Design review of the part built by this model. Coordinates are the model's own, in mm. A direction names the side the tool comes from. Round coordinates to 2 decimals unless told otherwise and drop trailing zeros. Order: outer loops, then holes, each group sorted by start corner. A loop starts at its lowest first (then second) coordinate and runs counter-clockwise, first axis right, second up. Notation, with made-up numbers: M 10,40 L 38,40 A24 ccw 38,73 Z; hole C 35,67 d2. An arc over 180 degrees is marked long. Write each question's results on one line, items separated by ' | '. Start each with the question number.
Item 1: The part is to be moulded in two halves that separate along Y. For faces 1 (the flat face through (-1, 1.5, 6)), 2 (the cylindrical face through (51.64, -2.6, 4.31)), 3 (the flat face through (-1, 0, 2)), 4 (the cylindrical face through (-51.64, 2.6, 4.19)), say which applies: +Y half, -Y half, draft (parallel to the pull), parting line (faces both ways), or undercut.
Item 2: Wall thickness on line 1 (Y direction, x = -6, z = 3.25); line 2 (X direction, y = -0.75, z = 6); line 3 (Z direction, x = -46, y = 0.25): over which ranges is each line inside the solid? List them lowest first. Write a range as [from, to].
Item 3: Clearance check with a flat-ended pin moving along its axis: pin 1 (1.5 mm diameter, centred on x = -1, y = -0.5, fed in from +Z). State where the tip first meets the part, or that it passes through.
Item 4: Machinability: for faces 5 (the cylindrical face through (-51.64, -2.6, 4.31)), 6 (the flat face through (1, -1.5, 6)), which of the approach directions +Z, -Z, +X, -X, +Y, -Y give a long, thin tool a straight path to every point of the face, cutting with its end or side? Answer none if there is none.
Item 5: Take a section at B-B, the plane x = -31. Write out the cut boundary in (y, z).
Item 6: Take a section at A-A, the plane z = 7.5. Write out the cut boundary in (x, y).
```python
from build123d import *

# Parameters (mm, degrees)
F0_W     = 105
F0_H     = 7
F1_DEPTH = 2
F2_DEPTH = 10
F3_R     = 3
F4_R     = 1.5


with BuildPart() as f1:
    # F0 (on Top) → F1 (new body)
    with BuildSketch(Plane.XY):
        Rectangle(F0_W, F0_H)
        with BuildLine():
            ThreePointArc((-50.5, 0), (-50.0606601718, 1.0606601718), (-49, 1.5))
            Line((-49, 1.5), (49, 1.5))
            ThreePointArc((49, 1.5), (50.0606601718, 1.0606601718), (50.5, 0))
            ThreePointArc((50.5, 0), (50.0606601718, -1.0606601718), (49, -1.5))
            Line((49, -1.5), (-49, -1.5))
            ThreePointArc((-49, -1.5), (-50.0606601718, -1.0606601718), (-50.5, 0))
        make_face(mode=Mode.SUBTRACT)
        with BuildLine():
            Line((49, 1.5), (-49, 1.5))
            ThreePointArc((-49, 1.5), (-50.0606601718, 1.0606601718), (-50.5, 0))
            ThreePointArc((-50.5, 0), (-50.0606601718, -1.0606601718), (-49, -1.5))
            Line((-49, -1.5), (49, -1.5))
            ThreePointArc((49, -1.5), (50.0606601718, -1.0606601718), (50.5, 0))
            ThreePointArc((50.5, 0), (50.0606601718, 1.0606601718), (49, 1.5))
        make_face()
    extrude(amount=F1_DEPTH)

    # F0 (on Top) → F2 (join)
    with BuildSketch(Plane.XY):
        Rectangle(F0_W, F0_H)
        with BuildLine():
            ThreePointArc((-50.5, 0), (-50.0606601718, 1.0606601718), (-49, 1.5))
            Line((-49, 1.5), (49, 1.5))
            ThreePointArc((49, 1.5), (50.0606601718, 1.0606601718), (50.5, 0))
            ThreePointArc((50.5, 0), (50.0606601718, -1.0606601718), (49, -1.5))
            Line((49, -1.5), (-49, -1.5))
            ThreePointArc((-49, -1.5), (-50.0606601718, -1.0606601718), (-50.5, 0))
        make_face(mode=Mode.SUBTRACT)
    extrude(amount=F2_DEPTH)

    # F3
    f3_edges = [f1.edges().sort_by_distance(p)[0] for p in [
        (-52.5, -3.5, 5),
        (52.5, -3.5, 5),
        (52.5, 3.5, 5),
        (-52.5, 3.5, 5),
    ]]
    fillet(f3_edges, radius=F3_R)

    # F4
    f4_edges = [f1.edges().sort_by_distance(p)[0] for p in [
        (0, 3.5, 10),
    ]]
    fillet(f4_edges, radius=F4_R)


solid = f1.part
```
Results list:
1) face 1: undercut | face 2: -Y half | face 3: undercut | face 4: +Y half
2) line 1: [-3.5, -1.5], [1.5, 3.5] | line 2: [-52.49, -50.3], [50.3, 52.49] | line 3: [0, 2]
3) pin 1: z = 2
4) face 5: +Z, -Z, -X, -Y | face 6: +Z
5) outline: M -3.5,0 L 3.5,0 L 3.5,8.5 A1.5 ccw 2,10 L 1.5,10 L 1.5,2 L -1.5,2 L -1.5,10 L -2,10 A1.5 ccw -3.5,8.5 Z
6) outline: M -52.5,-0.5 A3 ccw -49.5,-3.5 L 49.5,-3.5 A3 ccw 52.5,-0.5 L 52.5,0.5 A3 ccw 49.5,3.5 L -49.5,3.5 A3 ccw -52.5,0.5 Z; hole M -49,-1.5 L 49,-1.5 A1.5 ccw 49,1.5 L -49,1.5 A1.5 ccw Z
